from build123d import *

# Parameters (mm, degrees)
SKETCH1_R           = 2.15
SKETCH1_R_2         = 6.5
SKETCH1_W           = 25
SKETCH1_H           = 6
BOSS_EXTRUDE1_DEPTH = 6


with BuildPart() as part:
    # Sketch1 → Boss-Extrude1 (new body)
    with BuildSketch(Plane(origin=(0, 0, 0), x_dir=(1, 0, 0), z_dir=(0, 1, 0))):
        with BuildLine():
            Line((-10, 60), (10, 60))
            ThreePointArc((10, 60), (17.071067812, 57.071067812), (20, 50))
            Line((20, 50), (20, -60))
            Line((20, -60), (13, -60))
            Line((13, -60), (13, -66))
            Line((13, -66), (2, -66))
            Line((2, -66), (2, -58))
            Line((2, -58), (3.5, -58))
            Line((3.5, -58), (3.5, -54.8))
            Line((3.5, -54.8), (2, -54.8))
            Line((2, -54.8), (2, -50.8))
            Line((2, -50.8), (-2, -50.8))
            Line((-2, -50.8), (-2, -54.8))
            Line((-2, -54.8), (-3.5, -54.8))
            Line((-3.5, -54.8), (-3.5, -58))
            Line((-3.5, -58), (-2, -58))
            Line((-2, -58), (-2, -66))
            Line((-2, -66), (-13, -66))
            Line((-13, -66), (-13, -60))
            Line((-13, -60), (-20, -60))
            Line((-20, -60), (-20, 50))
            ThreePointArc((-20, 50), (-17.071067812, 57.071067812), (-10, 60))
        make_face()
        with Locations((4.85, 55)):
            Circle(SKETCH1_R, mode=Mode.SUBTRACT)
        with Locations((0, 41)):
            Circle(SKETCH1_R_2, mode=Mode.SUBTRACT)
        with Locations((4.85, 7)):
            Circle(SKETCH1_R, mode=Mode.SUBTRACT)
        with Locations((-4.85, 55)):
            Circle(SKETCH1_R, mode=Mode.SUBTRACT)
        with Locations((-4.85, 7)):
            Circle(SKETCH1_R, mode=Mode.SUBTRACT)
        with Locations((0, -4)):
            Rectangle(SKETCH1_W, SKETCH1_H, mode=Mode.SUBTRACT)
    extrude(amount=-BOSS_EXTRUDE1_DEPTH)


solid = part.part
Read the model definition and answer for the solid it produces. Units are mm, in the model's axes. A direction names the side the tool comes from. Give positions to 0.01 mm unless a question says otherwise; leave off trailing zeros. Write each loop counter-clockwise with the first axis right and the second up, starting at its lowest first coordinate (ties: lowest second). Pieces come first, ordered by that corner, then holes. Notation, with made-up numbers: (-16.5, 30.25) - (-1.5, 30.25) arc R24 cw to (-1.5, 59.25) - close; hole circle Ø5 at (68.25, -2). An arc over 180 degrees is marked (long way). Return JSON: item names as keys, results as strings.
Q1. For a pull along Z with two mould halves and no side action, classify faces 1 (the face through (-2, -3, 62)), 2 (the face through (8, -3, 66)), 3 (the face through (-5.13, -2.96, -9.13)) as released by +Z, released by -Z, zero draft, split by the parting line, or undercut.
Reply:
{"face 1": "zero draft", "face 2": "released by +Z", "face 3": "undercut"}
Q2. For faces 4 (the face through (-13, -3, 63)), 5 (the face through (-2, -3, 53)), 6 (the face through (13, -3, 63)), 7 (the face through (0, -3, 1)), 8 (the face through (16.99, -2.96, -57.15)), determine the directions among +Z, -Z, +X, -X, +Y, -Y from which every point of the face is accessible in a straight line to the end or side of a thin tool.
Reply:
{"face 4": "+Z, -X, +Y, -Y", "face 5": "+Z, +Y, -Y", "face 6": "+Z, +X, +Y, -Y", "face 7": "+Y, -Y", "face 8": "-Z, +X, +Y, -Y"}
Q3. A cutting plane is placed at D-D, the plane z = -7. Determine the outline of the cut face in (x, y), and give its area (3 significant figures).
Reply:
{"outline": "(-20, -6) - (-7, -6) - (-7, 0) - (-20, 0) - close; (-2.7, -6) - (2.7, -6) - (2.7, 0) - (-2.7, 0) - close; (7, -6) - (20, -6) - (20, 0) - (7, 0) - close", "area": "188 mm²"}
Q4. A cutting plane is placed at C-C, the plane y = -3.3. Count the separate pieces of the cut face and the enclosed holes in it, and give its area (3 significant figures).
Reply:
{"separate pieces": "1", "enclosed holes": "6", "area": "4,500 mm²"}
Q5. A cutting plane is placed at A-A, the plane z = -41. Determine the outline of the cut face in (x, y), and give its area (3 significant figures).
Reply:
{"outline": "(-20, -6) - (-6.5, -6) - (-6.5, 0) - (-20, 0) - close; (6.5, -6) - (20, -6) - (20, 0) - (6.5, 0) - close", "area": "162 mm²"}
Q6. Given P1, Ø3, axis at y = -3.5, z = 63.5, coming from the +X side, flat-ended and moving along its own axis, determine where the tip first touches the part or whether it passes through.
Reply:
{"P1": "x = 13"}
Q7. Consider line 1 along Z through (x, y) = (-3, -1.8); line 2 along Z through (x, y) = (4.85, -4.25); line 3 along X through (y, z) = (-1.25, -7). Determine where each line is inside the solid, lowest interval first. Write a range as [from, to].
Reply:
{"line 1": "[-60, -56.1], [-53.9, -46.77], [-35.23, -8.1], [-5.9, 1], [7, 54.8], [58, 66]", "line 2": "[-60, -57.15], [-52.85, -45.33], [-36.67, -9.15], [-4.85, 1], [7, 66]", "line 3": "[-20, -7], [-2.7, 2.7], [7, 20]"}
Q8. A cutting plane is placed at B-B, the plane x = 0. Determine the outline of the cut face in (y, z), and give its area (3 significant figures).
Reply:
{"outline": "(-6, -60) - (0, -60) - (0, -47.5) - (-6, -47.5) - close; (-6, -34.5) - (0, -34.5) - (0, 1) - (-6, 1) - close; (-6, 7) - (0, 7) - (0, 50.8) - (-6, 50.8) - close", "area": "551 mm²"}
